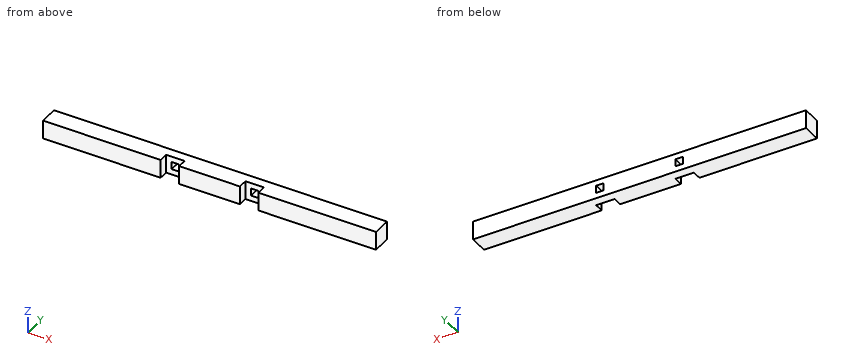
from build123d import *

# Parameters (mm, degrees)
SKETCH1_W           = 25
SKETCH1_H           = 25
BOSS_EXTRUDE1_DEPTH = 450
SKETCH2_W           = 10
SKETCH2_H           = 10
CUT_EXTRUDE1_DEPTH  = 452.386752132
SKETCH3_W           = 25
SKETCH3_H           = 25
CUT_EXTRUDE2_DEPTH  = 12.5


with BuildPart() as part:
    # Sketch1 → Boss-Extrude1 (new body)
    with BuildSketch(Plane(origin=(0, 0, 0), x_dir=(0, 0, -1), z_dir=(1, 0, 0))):
        with Locations((12.5, 12.5)):
            Rectangle(SKETCH1_W, SKETCH1_H)
    extrude(amount=BOSS_EXTRUDE1_DEPTH)

    # Sketch2 → Cut-Extrude1 (cut, through all)
    with BuildSketch(Plane(origin=(0, 25, 0), x_dir=(1, 0, 0), z_dir=(0, 1, 0))):
        with Locations((278.5, 12.5)):
            Rectangle(SKETCH2_W, SKETCH2_H)
        with Locations((171.5, 12.5)):
            Rectangle(SKETCH2_W, SKETCH2_H)
    extrude(amount=-CUT_EXTRUDE1_DEPTH, mode=Mode.SUBTRACT)

    # Sketch3 → Cut-Extrude2 (cut)
    with BuildSketch(Plane.XZ):
        with Locations((278.5, -12.5)):
            Rectangle(SKETCH3_W, SKETCH3_H)
        with Locations((171.5, -12.5)):
            Rectangle(SKETCH3_W, SKETCH3_H)
    extrude(amount=-CUT_EXTRUDE2_DEPTH, mode=Mode.SUBTRACT)


solid = part.part
CAD build for the part. Positions are in the model's coordinates, mm. Coordinates: 2 decimals unless noted, no trailing zeros. Order: outer loops, then holes, each group sorted by start corner. A loop starts at its lowest first (then second) coordinate and runs counter-clockwise, first axis right, second up.
Item 1: Band-saw the part on B-B on z = -13. List the corners of the cut face in (x, y).
Check sheet entries:
outline: (0, 0) - (159, 0) - (159, 12.5) - (166.5, 12.5) - (166.5, 25) - (0, 25) - close; (176.5, 12.5) - (184, 12.5) - (184, 0) - (266, 0) - (266, 12.5) - (273.5, 12.5) - (273.5, 25) - (176.5, 25) - close; (283.5, 12.5) - (291, 12.5) - (291, 0) - (450, 0) - (450, 25) - (283.5, 25) - close
Item 2: Drill centre lines: L1, parallel to X at y = 13.75, z = -14.75; L2, parallel to X at y = 8.5, z = -24; L3, parallel to Y at x = 275.5, z = -5. Where is each one in solid material? Low to high.
Check sheet entries:
L1: x = 0 to 166.5, 176.5 to 273.5, 283.5 to 450
L2: x = 0 to 159, 184 to 266, 291 to 450
L3: y = 12.5 to 25
Item 3: Band-saw the part on A-A on y = 4.75. List the corners of the cut face in (x, z).
Check sheet entries:
outline: (0, -25) - (159, -25) - (159, 0) - (0, 0) - close; (184, -25) - (266, -25) - (266, 0) - (184, 0) - close; (291, -25) - (450, -25) - (450, 0) - (291, 0) - close
Item 4: Pin check, flat tips, straight feed: pin 1 Ø12.5 at (x, z) = (171, -10) entering from -Y; pin 2 Ø11 at (x, y) = (278, 17) entering from +Z. Stop position of each tip, or through.
Check sheet entries:
pin 1: stops at y = 12.5
pin 2: stops at z = 0
